from build123d import *

# Parameters (mm, degrees)
F0_R     = 4
F0_R_2   = 3
F1_DEPTH = 25
F0_R_3   = 4.5
F2_DEPTH = 2
F5_D     = 3.4


with BuildPart() as f1:
    # F0 (on Top) → F1 (new body)
    with BuildSketch(Plane.XY):
        Circle(F0_R)
        Circle(F0_R_2, mode=Mode.SUBTRACT)
    extrude(amount=F1_DEPTH)

    # F0 (on Top) → F2 (join)
    with BuildSketch(Plane.XY):
        Circle(F0_R_3)
        Circle(F0_R, mode=Mode.SUBTRACT)
    extrude(amount=F2_DEPTH)

    # F5 (through all)
    with Locations(Plane.XZ.offset(4)):
        with Locations((0, 20)):
            Hole(F5_D / 2)


solid = f1.part
The model under review builds one solid part; all positions refer to its coordinate system, in mm. A direction names the side the tool comes from. Round coordinates to 2 decimals unless told otherwise and drop trailing zeros. Order: outer loops, then holes, each group sorted by start corner. A loop starts at its lowest first (then second) coordinate and runs counter-clockwise, first axis right, second up. Notation, with made-up numbers: (32.5, -37) -> (41.5, -37) arc R6 cw to (41.5, -32) -> close; hole circle Ø3 at (23, -30). An arc over 180 degrees is marked (long way). Use CSV: the item, a comma, the result in double quotes. Start each with the question number.
(1) Consider section A-A on x = 0. Write out the cut boundary in (y, z).
(2) Consider section D-D on z = 20. Write out the cut boundary in (x, y).
(3) Consider section C-C on x = -2.75. Write out the cut boundary in (y, z).
(4) Insertion check: pin 1 (1 mm diameter, centred on x = -3.5, z = 11, fed in from -Y); pin 2 (4 mm diameter, centred on x = 1, z = 13, fed in from -Y); pin 3 (1 mm diameter, centred on y = 0, z = 5.5, fed in from -X). Each pin has a flat end and moves straight along its axis. Give the tip position at first contact, or say it passes through.
(5) Tool access review of faces 1 (the face through (1.7, 3.25, 20.07)), 2 (the face through (1.846, -3.549, 13.339)): name each direction out of +Z, -Z, +X, -X, +Y, -Y from which nothing blocks a thin tool from reaching the whole face with its end or side.
(6) Consider section B-B on y = 0. Write out the cut boundary in (x, z), and give its area (3 significant figures).
(7) Wall thickness on probe 1 along Z at (x, y) = (0, -3.4); probe 2 along Z at (x, y) = (0.5, 4); probe 3 along X at (y, z) = (0.25, 2.5): over which ranges is each line inside the solid? List them lowest first. Write a range as from..to.
(8) Mouldability with a two-part tool opening along Z and no side actions: class faces 3 (the face through (1.35, -3.23, 18.97)), 4 (the face through (-0.59, 4.46, 0.99)), 5 (the face through (1, -3, 0)) as pulls with the +Z half, pulls with the -Z half, needs draft (parallel to the pull), parting line crosses it, or undercut.
Responses:
1,outline,"(-4.5, 0) -> (-3, 0) -> (-3, 18.3) -> (-4, 18.3) -> (-4, 2) -> (-4.5, 2) -> close; (-4, 21.7) -> (-3, 21.7) -> (-3, 25) -> (-4, 25) -> close; (3, 0) -> (4.5, 0) -> (4.5, 2) -> (4, 2) -> (4, 18.3) -> (3, 18.3) -> close; (3, 21.7) -> (4, 21.7) -> (4, 25) -> (3, 25) -> close"
2,outline,"(-1.7, -3.62) -> (-1.7, -2.47) arc R3 cw to (-1.7, 2.47) -> (-1.7, 3.62) arc R4 ccw to start; (1.7, -3.62) arc R4 ccw to (1.7, 3.62) -> (1.7, 2.47) arc R3 cw to (1.7, -2.47) -> close"
3,outline,"(-3.56, 0) -> (-1.2, 0) -> (-1.2, 25) -> (-2.9, 25) -> (-2.9, 2) -> (-3.56, 2) -> close; (1.2, 0) -> (3.56, 0) -> (3.56, 2) -> (2.9, 2) -> (2.9, 25) -> (1.2, 25) -> close"
4,pin 1,"y = -2.65"
4,pin 2,"y = -4"
4,pin 3,"x = -4"
5,face 1,"+Y, -Y"
5,face 2,"+Z"
6,outline,"(-4.5, 0) -> (-3, 0) -> (-3, 25) -> (-4, 25) -> (-4, 2) -> (-4.5, 2) -> close; (3, 0) -> (4.5, 0) -> (4.5, 2) -> (4, 2) -> (4, 25) -> (3, 25) -> close"
6,area,"52.0 mm²"
7,probe 1,"0..18.3, 21.7..25"
7,probe 2,"0..2"
7,probe 3,"-3.99..-2.99, 2.99..3.99"
8,face 3,"undercut"
8,face 4,"needs draft"
8,face 5,"pulls with the -Z half"
